```python
from build123d import *

# Parameters (mm, degrees)
F2_R     = 1.5
F4_DEPTH = 4.2


with BuildPart() as f1:
    # F0 (on Front) → F1 (revolve)
    with BuildSketch(Plane.XZ):
        Polygon((-11.8, 0), (-8.75, 0), (-8.05, 7), (-8.75, 14.1), (-12.3, 14.1), (-17.5, 12.2), (-17.5, 8.3), (-13, 8.3), (-13, 6), (-13.4, 6), align=None)
    revolve(axis=Axis((0, 0, 7.750909), (0, 0, 1)))

    # F2
    f2_edges = [f1.edges().sort_by_distance(p)[0] for p in [
        (8.75, 0, 14.1),
    ]]
    fillet(f2_edges, radius=F2_R)

    # F3 (on face) → F4 (join)
    with BuildSketch(Plane(origin=(0, 0, 8.3), x_dir=(1, 0, 0), z_dir=(0, 0, -1))):
        with BuildLine():
            ThreePointArc((-12.803808, -2.25), (-13, 0), (-12.803808, 2.25))
            Line((-12.803808, 2.25), (-16, 2.25))
            Line((-16, 2.25), (-16, -2.25))
            Line((-16, -2.25), (-12.803808, -2.25))
        make_face()
        with BuildLine():
            Line((16, 2.25), (12.803808, 2.25))
            ThreePointArc((12.803808, 2.25), (12.950859, 1.129269), (13, 0))
            ThreePointArc((13, 0), (12.950859, -1.129269), (12.803808, -2.25))
            Line((12.803808, -2.25), (16, -2.25))
            Line((16, -2.25), (16, 2.25))
        make_face()
        with BuildLine():
            ThreePointArc((13, 0), (12.950859, 1.129269), (12.803808, 2.25))
            Line((12.803808, 2.25), (12, 2.25))
            Line((12, 2.25), (12, -2.25))
            Line((12, -2.25), (12.803808, -2.25))
            ThreePointArc((12.803808, -2.25), (12.950859, -1.129269), (13, 0))
        make_face()
        with BuildLine():
            Line((-12, -2.25), (-12, 2.25))
            Line((-12, 2.25), (-12.803808, 2.25))
            ThreePointArc((-12.803808, 2.25), (-13, 0), (-12.803808, -2.25))
            Line((-12.803808, -2.25), (-12, -2.25))
        make_face()
    extrude(amount=F4_DEPTH)


solid = f1.part
```
The model under review builds one solid part; all positions refer to its coordinate system, in mm. A direction names the side the tool comes from. Give positions to 0.01 mm unless a question says otherwise; leave off trailing zeros. Order: outer loops, then holes, each group sorted by start corner. A loop starts at its lowest first (then second) coordinate and runs counter-clockwise, first axis right, second up. Notation, with made-up numbers: (75, 49) - (120, 49) arc R20 ccw to (120, 75) - close; hole circle Ø2 at (-7.5, 85). An arc over 180 degrees is marked (long way). Use CSV: the item, a comma, the result in double quotes. Start each with the question number.
Q1. We need section C-C, the plane z = 11. Write out the cut boundary in (x, y), and give its area (3 significant figures).
Q2. We need section B-B, the plane y = 0. Write out the cut boundary in (x, z), and give its area (3 significant figures).
Q3. Tool access review of faces 1 (the cylindrical face through (0, -13, 7)), 2 (the flat face through (-0.1, 13.2, 6)), 3 (the flat face through (-16, 0, 6)), 4 (the flat face through (16, 0, 6)): name each direction out of +Z, -Z, +X, -X, +Y, -Y from which nothing blocks a thin tool from reaching the whole face with its end or side.
Q4. The part is to be moulded in two halves that separate along Y. For faces 5 (the conical face through (-10.97, 4.55, 0.29)), 6 (the flat face through (-14, 0, 4.1)), 7 (the conical face through (-3.82, 7.34, 9.28)), say which applies: +Y half, -Y half, draft (parallel to the pull), parting line (faces both ways), or undercut.
Q5. We need section A-A, the plane x = 0. Write out the cut boundary in (y, z), and give its area (3 significant figures).
Q6. Clearance check with flat-ended pins moving along their axes: pin 1 Ø1.5 at (x, z) = (3, 2) entering from -Y; pin 2 Ø6 at (x, y) = (1, -7) entering from -Z; pin 3 Ø6 at (x, y) = (-11.5, 12.5) entering from +Z; pin 4 Ø1.3 at (y, z) = (-1, 6.5) entering from +X. State where each tip first meets the part, or that it passes through.
Q7. To check wall thickness, follow line 1 along Z through (x, y) = (-15, -5); line 2 along Y through (x, z) = (0, 3); line 3 along Y through (x, z) = (0.5, 11.5). State the ranges of each line that lie inside material, in increasing order. Write a range as [from, to].
Outcome:
1,outline,"circle Ø35 at (0, 0); hole circle Ø16.89 at (0, 0)"
1,area,"738 mm^2"
2,outline,"(-17.5, 8.3) - (-16, 8.3) - (-16, 4.1) - (-12.89, 4.1) - (-11.8, 0) - (-8.75, 0) - (-8.05, 7) - (-8.62, 12.75) arc R1.5 ccw to (-10.11, 14.1) - (-12.3, 14.1) - (-17.5, 12.2) - close; (8.05, 7) - (8.75, 0) - (11.8, 0) - (12.89, 4.1) - (16, 4.1) - (16, 8.3) - (17.5, 8.3) - (17.5, 12.2) - (12.3, 14.1) - (10.11, 14.1) arc R1.5 ccw to (8.62, 12.75) - close"
2,area,"191 mm^2"
3,face 1,"-Y"
3,face 2,"+Y"
3,face 3,"-Z, -X, +Y, -Y"
3,face 4,"-Z, +X, +Y, -Y"
4,face 5,"parting line"
4,face 6,"draft"
4,face 7,"undercut"
5,outline,"(-17.5, 8.3) - (-13, 8.3) - (-13, 6) - (-13.4, 6) - (-11.8, 0) - (-8.75, 0) - (-8.05, 7) - (-8.62, 12.75) arc R1.5 ccw to (-10.11, 14.1) - (-12.3, 14.1) - (-17.5, 12.2) - close; (8.05, 7) - (8.75, 0) - (11.8, 0) - (13.4, 6) - (13, 6) - (13, 8.3) - (17.5, 8.3) - (17.5, 12.2) - (12.3, 14.1) - (10.11, 14.1) arc R1.5 ccw to (8.62, 12.75) - close"
5,area,"166 mm^2"
6,pin 1,"stops at y = -12.23"
6,pin 2,"stops at z = 0"
6,pin 3,"stops at z = 13.48"
6,pin 4,"stops at x = 16"
7,line 1,"z = [8.3, 12.82]"
7,line 2,"y = [-12.6, -8.45], [8.45, 12.6]"
7,line 3,"y = [-17.49, -8.48], [8.48, 17.49]"
